Read the model definition and answer for the solid it produces. Units are mm, in the model's axes. Face numbers are marked on the shaded views. A direction names the side the tool comes from. Coordinates: 2 decimals unless noted, no trailing zeros. Order: outer loops, then holes, each group sorted by start corner. A loop starts at its lowest first (then second) coordinate and runs counter-clockwise, first axis right, second up. Notation, with made-up numbers: M 89,77 L 112,77 A15 ccw 112,87 Z; hole C 17,44 d5. An arc over 180 degrees is marked long. Write each question's results on one line, items separated by ' | '.
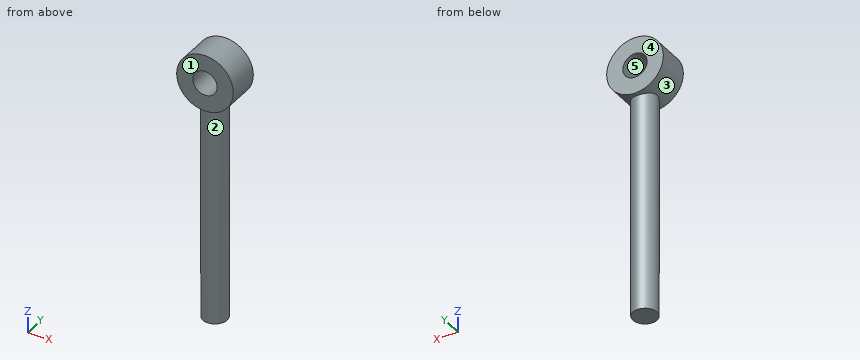
```python
from build123d import *

# Parameters (mm, degrees)
SKETCH_1_R           = 3
EXTRUDE_1_DEPTH      = 55
EXTRUDE_2_DEPTH      = 4
EXTRUDE_2_DEPTH_BACK = 4
SKETCH_3_R           = 7
SKETCH_4_R           = 3
CUT_EXTRUDE_1_DEPTH  = 69.825867351


with BuildPart() as part:
    # Sketch 1 → Extrude 1 (new body)
    with BuildSketch(Plane.XY):
        Circle(SKETCH_1_R)
    extrude(amount=EXTRUDE_1_DEPTH)

    # Sketch 3 → Extrude 2 (add, two sides: drawn at the far end of the back side and taken through both)
    with BuildSketch(Plane(origin=(0, 0, 0), x_dir=(1, 0, 0), z_dir=(0, 1, 0)).offset(-EXTRUDE_2_DEPTH_BACK)):
        with Locations(Location((0, -61, 0), (0, 0, 270))):
            Circle(SKETCH_3_R)
    extrude(amount=EXTRUDE_2_DEPTH + EXTRUDE_2_DEPTH_BACK)

    # Sketch 4 → Cut-Extrude 1 (cut, through all)
    with BuildSketch(Plane(origin=(0, 4, 0), x_dir=(1, 0, 0), z_dir=(0, 1, 0))):
        with Locations(Location((0, -61, 0), (0, 0, 270))):
            Circle(SKETCH_4_R)
    extrude(amount=-CUT_EXTRUDE_1_DEPTH, mode=Mode.SUBTRACT)


solid = part.part
```
(1) The part is cut by section B-B, the plane x = 0. Write down the section's boundary in (y, z).
Conclusion:
outline: M -4,54 L -3,54 L -3,0 L 3,0 L 3,54 L 4,54 L 4,58 L -4,58 Z; M -4,64 L 4,64 L 4,68 L -4,68 Z
(2) For the marked faces 1 and 2, determine the directions among +Z, -Z, +X, -X, +Y, -Y from which every point of the face is accessible in a straight line to the end or side of a thin tool.
Conclusion:
face 1: +Z, -Z, +X, -X, -Y | face 2: -Z
(3) The part is cut by section D-D, the plane z = 22. Write down the section's boundary in (x, y).
Conclusion:
outline: C 0,0 d6
(4) Given pin 1 (8 mm diameter, centred on x = -4.5, z = 18, fed in from +Y); pin 2 (2 mm diameter, centred on x = 2.5, y = 3, fed in from -Z); pin 3 (2 mm diameter, centred on x = 5, y = -1, fed in from -Z); pin 4 (1 mm diameter, centred on y = -2.5, z = 30.5, fed in from +X), each flat-ended and moving along its own axis, determine where each tip first touches the part or whether it passes through.
Conclusion:
pin 1: y = 2.96 | pin 2: z = 0 | pin 3: z = 55.26 | pin 4: x = 2.24
(5) The part is cut by section A-A, the plane z = 61. Write down the section's boundary in (x, y).
Conclusion:
outline: M -7,-4 L -3,-4 L -3,4 L -7,4 Z; M 3,-4 L 7,-4 L 7,4 L 3,4 Z
(6) The mould has two halves that part along X. Classify the marked faces 3, 4 and 5: pulls with the +X half, pulls with the -X half, needs draft (parallel to the pull), parting line crosses it, or undercut.
Conclusion:
face 3: parting line crosses it | face 4: needs draft | face 5: undercut
(7) The part is cut by section C-C, the plane y = 0. Write down the section's boundary in (x, z).
Conclusion:
outline: M -3,0 L 3,0 L 3,54.68 A7 ccw long -3,54.68 Z; hole C 0,61 d6
(8) Straight lines are drawn through the part: line 1 (X direction, y = 1.5, z = 61); line 2 (Y direction, x = -0.25, z = 27); line 3 (Z direction, x = -1.5, y = 2.5). For each, find the intervals that lie inside material, in ascending order.
Conclusion:
line 1: -7 to -3, 3 to 7 | line 2: -2.99 to 2.99 | line 3: 0 to 58.4, 63.6 to 67.84
